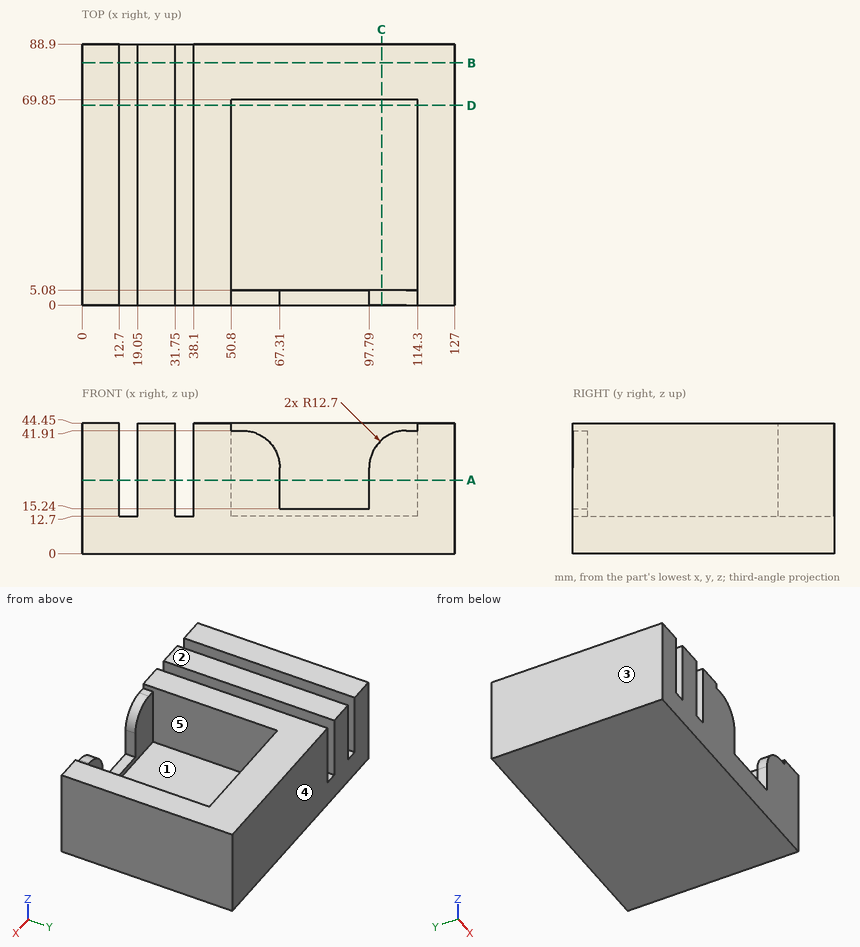
Check sheet for the drawn part. Datum: minimum x, y, z corner. Units: mm. A direction names the side the tool comes from. Round coordinates to 2 decimals unless told otherwise and drop trailing zeros. Order: outer loops, then holes, each group sorted by start corner. A loop starts at its lowest first (then second) coordinate and runs counter-clockwise, first axis right, second up.
1) Scan lines: line 1 (X direction, y = 59, z = 33); line 2 (X direction, y = 72, z = 32.5); line 3 (Y direction, x = 113, z = 22). Record each from-to range of solid material in increasing order.
2) Section check D-D (y = 68). Record the boundary of the cut face in (x, z), and give its area (3 significant figures).
3) Section check C-C (x = 102). Record the boundary of the cut face in (y, z), and give its area (3 significant figures).
4) Section check B-B (y = 82.5). Record the boundary of the cut face in (x, z), and give its area (3 significant figures).
5) Go/stop test with flat-tipped pins: pin 1 Ø4 at (x, y) = (88.5, 4) entering from +Z; pin 2 Ø10 at (x, y) = (97, 10.5) entering from +Z; pin 3 Ø3 at (x, y) = (53, 2) entering from +Z. Record where each tip stops, or that it passes through.
6) Mould release check, pull along X, two halves, no side actions. Record for the marked faces 1, 2 and 3: +X half, -X half, draft (parallel to the pull), parting line (faces both ways), or undercut.
7) Tool access check on the marked faces 4 and 5. Record the directions out of +Z, -Z, +X, -X, +Y, -Y that give a thin tool (end or side, any length) a straight path to the whole face; none if there is none.
8) Section check A-A (z = 25). Record the boundary of the cut face in (x, y).
Result:
1. line 1: x = 0 to 12.7, 19.05 to 31.75, 38.1 to 50.8, 114.3 to 127
1. line 2: x = 0 to 12.7, 19.05 to 31.75, 38.1 to 127
1. line 3: y = 0 to 5.08, 69.85 to 88.9
2. outline: (0, 0) - (127, 0) - (127, 44.45) - (114.3, 44.45) - (114.3, 12.7) - (50.8, 12.7) - (50.8, 44.45) - (38.1, 44.45) - (38.1, 12.7) - (31.75, 12.7) - (31.75, 44.45) - (19.05, 44.45) - (19.05, 12.7) - (12.7, 12.7) - (12.7, 44.45) - (0, 44.45) - close
2. area: 3,230 mm2
3. outline: (0, 0) - (88.9, 0) - (88.9, 44.45) - (69.85, 44.45) - (69.85, 12.7) - (5.08, 12.7) - (5.08, 38.66) - (0, 38.66) - close
3. area: 1,870 mm2
4. outline: (0, 0) - (127, 0) - (127, 44.45) - (38.1, 44.45) - (38.1, 12.7) - (31.75, 12.7) - (31.75, 44.45) - (19.05, 44.45) - (19.05, 12.7) - (12.7, 12.7) - (12.7, 44.45) - (0, 44.45) - close
4. area: 5,240 mm2
5. pin 1: stops at z = 15.24
5. pin 2: stops at z = 12.7
5. pin 3: stops at z = 41.91
6. face 1: undercut
6. face 2: draft
6. face 3: -X half
7. face 4: +Z, -Z, +X, -X, +Y
7. face 5: +Z
8. outline: (0, 0) - (12.7, 0) - (12.7, 88.9) - (0, 88.9) - close; (19.05, 0) - (31.75, 0) - (31.75, 88.9) - (19.05, 88.9) - close; (38.1, 0) - (67.31, 0) - (67.31, 5.08) - (50.8, 5.08) - (50.8, 69.85) - (114.3, 69.85) - (114.3, 5.08) - (97.79, 5.08) - (97.79, 0) - (127, 0) - (127, 88.9) - (38.1, 88.9) - close
